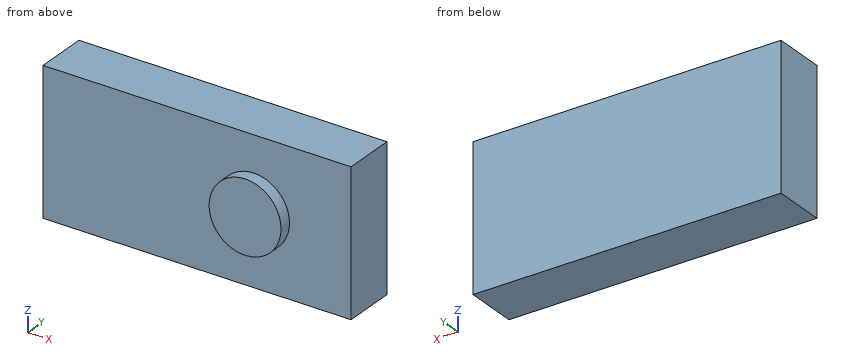
from build123d import *

# Parameters (mm, degrees)
SKETCH_2_W      = 60
SKETCH_2_H      = 28
EXTRUDE_1_DEPTH = 10.2
SKETCH_3_R      = 7
EXTRUDE_2_DEPTH = 2.4


with BuildPart() as part:
    # 草图2 → 凸台-拉伸1 (new body)
    with BuildSketch(Plane(origin=(0, 0, 0), x_dir=(1, 0, 0), z_dir=(0, 1, 0))):
        with Locations((10.280701754, -4.807017544)):
            Rectangle(SKETCH_2_W, SKETCH_2_H)
    extrude(amount=EXTRUDE_1_DEPTH)

    # 草图3 → 凸台-拉伸2 (add)
    with BuildSketch(Plane.XZ):
        with Locations((21.280701754, 4.807017544)):
            Circle(SKETCH_3_R)
    extrude(amount=EXTRUDE_2_DEPTH)


solid = part.part
Design review of the part built by this model. Coordinates are the model's own, in mm. Round coordinates to 2 decimals unless told otherwise and drop trailing zeros. Loops run counter-clockwise (first coordinate to the right, second up) from the corner with the lowest first, then second, coordinate; pieces in that order, holes last. Notation, with made-up numbers: M -38,7 L -23,7 A32 cw -23,36 Z; hole C -16.5,-20.75 d1. An arc over 180 degrees is marked long. Answer as a JSON object with one key per item and string values.
Item 1: We need section D-D on z = -4.75. Give the boundary of the cut face in (x, y), and give its area (3 significant figures).
Answer sheet:
{"outline": "M -19.72,0 L 40.28,0 L 40.28,10.2 L -19.72,10.2 Z", "area": "612 mm^2"}
Item 2: We need section B-B on z = 1. Give the boundary of the cut face in (x, y).
Answer sheet:
{"outline": "M -19.72,0 L 15.41,0 L 15.41,-2.4 L 27.15,-2.4 L 27.15,0 L 40.28,0 L 40.28,10.2 L -19.72,10.2 Z"}
Item 3: We need section C-C on y = -1.25. Give the boundary of the cut face in (x, z).
Answer sheet:
{"outline": "C 21.28,4.81 d14"}
Item 4: Wall thickness on L1, parallel to Y at x = 19, z = 17.75; L2, parallel to X at y = -1, z = 4.5; L3, parallel to X at y = -1.5, z = 0: over which ranges is each line inside the solid? List them lowest first. Write a range as from..to.
Answer sheet:
{"L1": "y = 0..10.2", "L2": "x = 14.29..28.27", "L3": "x = 16.19..26.37"}
Item 5: We need section A-A on x = 18.5. Give the boundary of the cut face in (y, z), and give its area (3 significant figures).
Answer sheet:
{"outline": "M -2.4,-1.62 L 0,-1.62 L 0,-9.19 L 10.2,-9.19 L 10.2,18.81 L 0,18.81 L 0,11.23 L -2.4,11.23 Z", "area": "316 mm^2"}
